```python
from build123d import *
from OCP.BRepFilletAPI import BRepFilletAPI_MakeChamfer

# Parameters (mm, degrees)
BOSS_EXTRUDE1_DEPTH = 5
HOLE1_D             = 4.917
CHAMFER1_SIZE       = 0.75
CHAMFER1_SIZE_2     = 0.433012702
CHAMFER2_SIZE       = 0.5415


with BuildPart() as part:
    # Sketch1 → Boss-Extrude1 (new body)
    with BuildSketch(Plane(origin=(-2.5, 0, 0), x_dir=(0, -1, 0), z_dir=(-1, 0, 0))):
        with BuildLine():
            Line((5.749854105, 0.040960553), (2.910399932, 4.959039447))
            ThreePointArc((2.910399932, 4.959039447), (2.875, 4.979646072), (2.839454173, 5))
            Line((2.839454173, 5), (-2.839454173, 5))
            ThreePointArc((-2.839454173, 5), (-2.875, 4.979646072), (-2.910399932, 4.959039447))
            Line((-2.910399932, 4.959039447), (-5.749854105, 0.040960553))
            ThreePointArc((-5.749854105, 0.040960553), (-5.75, 0), (-5.749854105, -0.040960553))
            Line((-5.749854105, -0.040960553), (-2.910399932, -4.959039447))
            ThreePointArc((-2.910399932, -4.959039447), (-2.875, -4.979646072), (-2.839454173, -5))
            Line((-2.839454173, -5), (2.839454173, -5))
            ThreePointArc((2.839454173, -5), (2.875, -4.979646072), (2.910399932, -4.959039447))
            Line((2.910399932, -4.959039447), (5.749854105, -0.040960553))
            ThreePointArc((5.749854105, -0.040960553), (5.75, 0), (5.749854105, 0.040960553))
        make_face()
    extrude(amount=-BOSS_EXTRUDE1_DEPTH)

    # Hole1 (through all)
    with Locations(Plane.ZY.offset(2.5)):
        with Locations((0, 0)):
            Hole(HOLE1_D / 2)

    # Chamfer1
    chamfer1_edges_1 = [part.edges().sort_by_distance(p)[0] for p in [
        (-2.5, -5.75, 0),
    ]]
    chamfer1_side_1 = [part.faces().sort_by_distance(p)[0] for p in [
        (-2.5, -5.741339746, 0),
    ]]
    chamfer1_edges_2 = [part.edges().sort_by_distance(p)[0] for p in [
        (-2.5, 5.75, 0),
    ]]
    chamfer1_side_2 = [part.faces().sort_by_distance(p)[0] for p in [
        (-2.491339746, 5.75, 0),
    ]]
    chamfer1_edges_3 = [part.edges().sort_by_distance(p)[0] for p in [
        (-2.5, 0, -5),
    ]]
    chamfer1_side_3 = [part.faces().sort_by_distance(p)[0] for p in [
        (-2.5, 0, -4.991339746),
    ]]
    chamfer1_edges_4 = [part.edges().sort_by_distance(p)[0] for p in [
        (-2.5, -2.875, -4.979646072),
    ]]
    chamfer1_side_4 = [part.faces().sort_by_distance(p)[0] for p in [
        (-2.5, -2.870669873, -4.972146072),
    ]]
    chamfer1_edges_5 = [part.edges().sort_by_distance(p)[0] for p in [
        (-2.5, 2.875, 4.979646072),
    ]]
    chamfer1_side_5 = [part.faces().sort_by_distance(p)[0] for p in [
        (-2.5, 2.870669873, 4.972146072),
    ]]
    chamfer1_edges_6 = [part.edges().sort_by_distance(p)[0] for p in [
        (-2.5, -2.875, 4.979646072),
    ]]
    chamfer1_side_6 = [part.faces().sort_by_distance(p)[0] for p in [
        (-2.5, -2.870669873, 4.972146072),
    ]]
    chamfer1 = BRepFilletAPI_MakeChamfer(part.part.solid().wrapped)
    for e in chamfer1_edges_1:
        chamfer1.Add(CHAMFER1_SIZE - 0.0001, CHAMFER1_SIZE_2 - 0.0001, e.wrapped, chamfer1_side_1[0].wrapped)
    for e in chamfer1_edges_2:
        chamfer1.Add(CHAMFER1_SIZE_2 - 0.0001, CHAMFER1_SIZE - 0.0001, e.wrapped, chamfer1_side_2[0].wrapped)
    for e in chamfer1_edges_3:
        chamfer1.Add(CHAMFER1_SIZE - 0.0001, CHAMFER1_SIZE_2 - 0.0001, e.wrapped, chamfer1_side_3[0].wrapped)
    for e in chamfer1_edges_4:
        chamfer1.Add(CHAMFER1_SIZE - 0.0001, CHAMFER1_SIZE_2 - 0.0001, e.wrapped, chamfer1_side_4[0].wrapped)
    for e in chamfer1_edges_5:
        chamfer1.Add(CHAMFER1_SIZE - 0.0001, CHAMFER1_SIZE_2 - 0.0001, e.wrapped, chamfer1_side_5[0].wrapped)
    for e in chamfer1_edges_6:
        chamfer1.Add(CHAMFER1_SIZE - 0.0001, CHAMFER1_SIZE_2 - 0.0001, e.wrapped, chamfer1_side_6[0].wrapped)
    add(Compound.cast(chamfer1.Shape()), mode=Mode.REPLACE)  # a hair under: the kernel refuses the full size

    # Chamfer2
    chamfer2_edges = [part.edges().sort_by_distance(p)[0] for p in [
        (-2.5, 0, 2.4585),
        (2.5, 0, 2.4585),
    ]]
    chamfer(chamfer2_edges, length=CHAMFER2_SIZE)


solid = part.part
```
Can you work these out from the model? Positions are in its coordinate system, mm. Give positions to 0.01 mm unless a question says otherwise; leave off trailing zeros. Order: outer loops, then holes, each group sorted by start corner. A loop starts at its lowest first (then second) coordinate and runs counter-clockwise, first axis right, second up. Notation, with made-up numbers: (38.5, 79.5) - (59.5, 79.5) arc R12 cw to (59.5, 99.5) - close; hole circle Ø1 at (-17, -6.5). An arc over 180 degrees is marked (long way). Use a Markdown table: item, result. Add a question column.
Q1. Please list where these lines run through material, in increasing order: line 1 along Y through (x, z) = (-1.05, 0); line 2 along Z through (x, y) = (0.4, 2.25); line 3 along Y through (x, z) = (-1.6, 0.5).
Q2. If we section it at A-A on x = 1.1: Write out the boundary of the cut face in (y, z), plus the area to 3 significant figures.
Q3. If we mould it in two halves opening along Y, with no side actions, what happens to faces 1 (the flat face through (-2.5, -2.2, 2.5)), 2 (the conical face through (-2.38, -5.21, -0.01)), 3 (the cylindrical face through (0.027, 0.738, -2.345))? For each: released by +Y, released by -Y, zero draft, split by the parting line, or undercut.
Q4. I'm going to push a flat-ended pin straight in: pin 1 (2 mm diameter, centred on x = -0.5, z = -2.5, fed in from -Y). Where does the tip first touch, or does it pass through?
Answers follow:
| question | item | result |
|---|---|---|
| 1 | line 1 | y = -5.75 to -2.46, 2.46 to 5.75 |
| 1 | line 2 | z = -5 to -0.99, 0.99 to 5 |
| 1 | line 3 | y = -5.48 to -2.41, 2.41 to 5.48 |
| 2 | outline | (-5.75, -0.04) - (-2.91, -4.96) arc R5.75 ccw to (-2.84, -5) - (2.84, -5) arc R5.75 ccw to (2.91, -4.96) - (5.75, -0.04) arc R5.75 ccw to (5.75, 0.04) - (2.91, 4.96) arc R5.75 ccw to (2.84, 5) - (-2.84, 5) arc R5.75 ccw to (-2.91, 4.96) - (-5.75, 0.04) arc R5.75 ccw to start; hole circle Ø4.92 at (0, 0) |
| 2 | area | 67.6 mm^2 |
| 3 | face 1 | zero draft |
| 3 | face 2 | released by -Y |
| 3 | face 3 | undercut |
| 4 | pin 1 | stops at y = -4.91 |
